from build123d import *

# Parameters (mm, degrees)
SKETCH1_W           = 40
SKETCH1_H           = 5
BOSS_EXTRUDE1_DEPTH = 4
SKETCH2_R           = 1.525
CUT_EXTRUDE1_DEPTH  = 41.509258201
SKETCH3_W           = 10
SKETCH3_H           = 2
SKETCH3_W_2         = 8.5
CUT_EXTRUDE2_DEPTH  = 41.509258201
FILLET1_R           = 0.75


with BuildPart() as part:
    # Sketch1 → Boss-Extrude1 (new body)
    with BuildSketch(Plane(origin=(0, 0, 0), x_dir=(1, 0, 0), z_dir=(0, 1, 0))):
        with Locations((20, 2.5)):
            Rectangle(SKETCH1_W, SKETCH1_H)
    extrude(amount=BOSS_EXTRUDE1_DEPTH)

    # Sketch2 → Cut-Extrude1 (cut, through all)
    with BuildSketch(Plane(origin=(0, 4, 0), x_dir=(1, 0, 0), z_dir=(0, 1, 0))):
        with Locations(Location((5, 2.5, 0), (0, 0, 270))):
            Circle(SKETCH2_R)
        with Locations(Location((35, 2.5, 0), (0, 0, 90))):
            Circle(SKETCH2_R)
    extrude(amount=-CUT_EXTRUDE1_DEPTH, mode=Mode.SUBTRACT)

    # Sketch3 → Cut-Extrude2 (cut, through all)
    with BuildSketch(Plane(origin=(0, 0, -5), x_dir=(-1, 0, 0), z_dir=(0, 0, -1))):
        with Locations((-35, 2)):
            Rectangle(SKETCH3_W, SKETCH3_H)
        with Locations((-24.75, 2)):
            Rectangle(SKETCH3_W_2, SKETCH3_H)
        with Locations((-15.25, 2)):
            Rectangle(SKETCH3_W_2, SKETCH3_H)
        with Locations((-5, 2)):
            Rectangle(SKETCH3_W, SKETCH3_H)
    extrude(amount=-CUT_EXTRUDE2_DEPTH, mode=Mode.SUBTRACT)

    # Fillet1
    fillet1_edges = [part.edges().sort_by_distance(p)[0] for p in [
        (30, 1, -2.5),
        (30, 3, -2.5),
        (29, 1, -2.5),
        (29, 3, -2.5),
        (20.5, 3, -2.5),
        (20.5, 1, -2.5),
        (19.5, 3, -2.5),
        (11, 3, -2.5),
        (11, 1, -2.5),
        (19.5, 1, -2.5),
        (10, 3, -2.5),
        (10, 1, -2.5),
    ]]
    fillet(fillet1_edges, radius=FILLET1_R)


solid = part.part
Work out the finished part from the listing and answer in its coordinate system (mm). A direction names the side the tool comes from. Round coordinates to 2 decimals unless told otherwise and drop trailing zeros. Write each loop counter-clockwise with the first axis right and the second up, starting at its lowest first coordinate (ties: lowest second). Pieces come first, ordered by that corner, then holes. Notation, with made-up numbers: M 4.25,43.5 L 12.25,43.5 A14 ccw 12.25,48.5 Z; hole C 84,62 d9. An arc over 180 degrees is marked long. Use a Markdown table: item, result.
1) Determine the mould class of faces 6 (the face through (15, 1, -3)), 7 (the face through (0, 0.5, -2.5)), 8 (the face through (20, 4, -3)) for opening direction Y: pulls with the +Y half, pulls with the -Y half, needs draft (parallel to the pull), parting line crosses it, or undercut.
Taken from the geometry:
| item | result |
|---|---|
| face 6 | undercut |
| face 7 | needs draft |
| face 8 | pulls with the +Y half |
2) Flat-ended cylindrical pins translate along their axes: pin 1 (1.5 mm diameter, centred on x = 5.5, z = -3, fed in from -Y); pin 2 (2.5 mm diameter, centred on x = 14.5, z = -2.5, fed in from -Y). Find the tip coordinate at first contact, or state that the pin passes through.
Taken from the geometry:
| item | result |
|---|---|
| pin 1 | passes through |
| pin 2 | stops at y = 0 |
3) The part is cut by section A-A on x = 35. Give the vertices of the cut face in (y, z) (3 decimals), plus the area to 3 significant figures.
Taken from the geometry:
| item | result |
|---|---|
| outline | M 0,-5 L 1,-5 L 1,-4.025 L 0,-4.025 Z; M 0,-0.975 L 1,-0.975 L 1,0 L 0,0 Z; M 3,-5 L 4,-5 L 4,-4.025 L 3,-4.025 Z; M 3,-0.975 L 4,-0.975 L 4,0 L 3,0 Z |
| area | 3.90 mm2 |
4) Consider line 1 (X direction, y = 0.85, z = -2.5) (3 decimals); line 2 (Y direction, x = 24, z = -0.75); line 3 (X direction, y = 1.8, z = -3.9). Determine where each line is inside the solid, lowest interval first. Write a range as [from, to].
Taken from the geometry:
| item | result |
|---|---|
| line 1 | x = [0, 3.475], [6.525, 33.475], [36.525, 40] |
| line 2 | y = [0, 1], [3, 4] |
| line 3 | x = [10, 11], [19.5, 20.5], [29, 30] |
5) Which of the six approach directions +Z, -Z, +X, -X, +Y, -Y give full straight-line access (tool end or side, diameter ignored) to faces 1 (the face through (4, 1, -4)), 2 (the face through (36.49, 0.51, -2.17)), 3 (the face through (25, 1, -3)), 4 (the face through (36, 1, -4)), 5 (the face through (20, 0, -3))?
Taken from the geometry:
| item | result |
|---|---|
| face 1 | +Z, -Z, -X |
| face 2 | +Y, -Y |
| face 3 | +Z, -Z |
| face 4 | +Z, -Z, +X |
| face 5 | +Z, -Z, +X, -X, -Y |
6) The part is cut by section B-B on z = -2.5. State how many separate pieces and enclosed holes the cut face has, plus the area to 3 significant figures.
Taken from the geometry:
| item | result |
|---|---|
| separate pieces | 5 |
| enclosed holes | 2 |
| area | 75.2 mm2 |
